from build123d import *

# Parameters (mm, degrees)
F1_DEPTH      = 15
F1_DEPTH_BACK = 15
F2_R          = 5
F4_DEPTH      = 25.0010001
F5_SIZE       = 1
F6_DEPTH      = 17


with BuildPart() as f1:
    # F0 (on Front) → F1 (new body, two sides)
    with BuildSketch(Plane.XZ) as f1_sk:
        with BuildLine():
            Line((10.947347623, 25), (-25, 25))
            Line((-25, 25), (-25, -25))
            Line((-25, -25), (10.947347623, -25))
            add(Edge.make_bspline(
                [(10.947347623, -25), (6.7776464895, -22.7393775974), (2.7889229832, -19.0392534951), (0, -15)],
                knots=[0.6583166498, 0.6583166498, 0.6583166498, 0.6583166498, 0.7610943584, 0.7610943584, 0.7610943584, 0.7610943584], degree=3))
            ThreePointArc((0, -15), (-15, 0), (0, 15))
            add(Edge.make_bspline(
                [(0, 15), (2.7889229832, 19.0392534951), (6.7776464895, 22.7393775974), (10.947347623, 25)],
                knots=[0, 0, 0, 0, 0.1027777086, 0.1027777086, 0.1027777086, 0.1027777086], degree=3))
        make_face()
    extrude(amount=-F1_DEPTH)
    extrude(f1_sk.sketch, amount=F1_DEPTH_BACK)

    # F2
    f2_edges = [f1.edges().sort_by_distance(p)[0] for p in [
        (-25, 0, 25),
        (-25, 0, -25),
    ]]
    fillet(f2_edges, radius=F2_R)

    # F3 (on Right) → F4 (cut, through all)
    with BuildSketch(Plane.YZ):
        with BuildLine():
            ThreePointArc((2, -1.5), (2.3717082451, -0.790569415), (2.5, 0))
            ThreePointArc((2.5, 0), (2.3717082451, 0.790569415), (2, 1.5))
            Line((2, 1.5), (-2, 1.5))
            ThreePointArc((-2, 1.5), (-2.5, 0), (-2, -1.5))
            Line((-2, -1.5), (2, -1.5))
        make_face()
        with BuildLine():
            ThreePointArc((-2, -1.5), (0, -2.5), (2, -1.5))
            Line((2, -1.5), (-2, -1.5))
        make_face()
        with BuildLine():
            Line((-2, 1.5), (2, 1.5))
            ThreePointArc((2, 1.5), (0, 2.5), (-2, 1.5))
        make_face()
    extrude(amount=-F4_DEPTH, mode=Mode.SUBTRACT)

    # F5
    f5_edges = [f1.edges().sort_by_distance(p)[0] for p in [
        (-25, -2, -1.5),
    ]]
    chamfer(f5_edges, length=F5_SIZE)

    # F3 (on Right) → F6 (cut)
    with BuildSketch(Plane.YZ):
        with BuildLine():
            ThreePointArc((2, 1.5), (2.3717082451, 0.790569415), (2.5, 0))
            ThreePointArc((2.5, 0), (2.3717082451, -0.790569415), (2, -1.5))
            Line((2, -1.5), (15, -1.5))
            Line((15, -1.5), (15, 1.5))
            Line((15, 1.5), (2, 1.5))
        make_face()
        with BuildLine():
            ThreePointArc((-2, -1.5), (-2.5, 0), (-2, 1.5))
            Line((-2, 1.5), (-15, 1.5))
            Line((-15, 1.5), (-15, -1.5))
            Line((-15, -1.5), (-2, -1.5))
        make_face()
    extrude(amount=-F6_DEPTH, mode=Mode.SUBTRACT)


solid = f1.part
The listing builds one solid part. Answer for the finished solid, in the listing's coordinates (mm). A direction names the side the tool comes from. Coordinates: 2 decimals unless noted, no trailing zeros. Loops run counter-clockwise (first coordinate to the right, second up) from the corner with the lowest first, then second, coordinate; pieces in that order, holes last.
1) Flat-ended cylindrical pins translate along their axes: pin 1 Ø4 at (y, z) = (0, 0) entering from -X; pin 2 Ø3.5 at (y, z) = (-6, -0.5) entering from +X; pin 3 Ø10 at (y, z) = (-3.5, 10.5) entering from +X; pin 4 Ø0.9 at (y, z) = (8.5, 0.5) entering from +X. Find the tip coordinate at first contact, or state that the pin passes through.
2) A tool of negligible diameter and unlimited length cuts with its end or side. For faces 5 (the face through (-16, 9, 1.5)), 6 (the face through (-23, 0, -24)), from which of +Z, -Z, +X, -X, +Y, -Y can it reach the whole face along a straight path? Write none if from no direction.
3) Find the intervals of material crossed by L1, parallel to Y at x = -21, z = 0; L2, parallel to Z at x = -0.5, y = 8; L3, parallel to Z at x = -15, y = -11, in increasing order.
4) Find section A-A on x = -9. Write down the section's boundary in (y, z).
5) Find section B-B on x = -2.5. Write down the section's boundary in (y, z).
6) Determine the mould class of faces 1 (the face through (-15, -15, 6)), 2 (the face through (-4, 0, 25)), 3 (the face through (-16, 8, -1.5)), 4 (the face through (-5, 0, -25)) for opening direction Z: pulls with the +Z half, pulls with the -Z half, needs draft (parallel to the pull), parting line crosses it, or undercut.
Values:
1. pin 1: passes through
1. pin 2: stops at x = -14.83
1. pin 3: stops at x = 0.35
1. pin 4: stops at x = -17
2. face 5: +X, +Y, -Y
2. face 6: -Z, -X, +Y, -Y
3. L1: y = -15 to -2.5, 2.5 to 15
3. L2: z = -25 to -14.99, 14.99 to 25
3. L3: z = -25 to -1.5, 1.5 to 25
4. outline: (-15, -25) - (15, -25) - (15, -12) - (-15, -12) - close; (-15, 12) - (15, 12) - (15, 25) - (-15, 25) - close
5. outline: (-15, -25) - (15, -25) - (15, -14.79) - (-15, -14.79) - close; (-15, 14.79) - (15, 14.79) - (15, 25) - (-15, 25) - close
6. face 1: needs draft
6. face 2: pulls with the +Z half
6. face 3: undercut
6. face 4: pulls with the -Z half
